The listing builds one solid part. Answer for the finished solid, in the listing's coordinates (mm). A direction names the side the tool comes from. Give positions to 0.01 mm unless a question says otherwise; leave off trailing zeros. Write each loop counter-clockwise with the first axis right and the second up, starting at its lowest first coordinate (ties: lowest second). Pieces come first, ordered by that corner, then holes. Notation, with made-up numbers: (87.25, 71.5) - (114.25, 71.5) arc R19 ccw to (114.25, 87.5) - close; hole circle Ø6 at (67.5, 79.25). An arc over 180 degrees is marked (long way). One line per question, with ' | ' between items. Start each with the question number.
1. Given P1, Ø1, axis at x = -3.5, z = 51.5, coming from the -Y side; P2, Ø6, axis at y = 8.5, z = 20, coming from the +X side; P3, Ø1.5, axis at y = -5, z = 85, coming from the +X side; P4, Ø10, axis at y = -2.5, z = 70.5, coming from the +X side, each flat-ended and moving along its own axis, determine where each tip first touches the part or whether it passes through.
2. Find the intervals of material crossed by L1, parallel to Z at x = -2, y = -2; L2, parallel to Y at x = -3, z = 68; L3, parallel to X at y = 0, z = 31.5, in increasing order. Write a range as from..to.
3. For faces 1 (the face through (-2.4, -1.8, 98)), 2 (the face through (-3, -2, 100)), determine the directions among +Z, -Z, +X, -X, +Y, -Y from which every point of the face is accessible in a straight line to the end or side of a thin tool.
4. The mould has two halves that part along X. Classify faces 3 (the face through (-1.08, 4.88, 46.75)), 4 (the face through (0, 0, 96)), 5 (the face through (0, 0, 0)): +X half, -X half, draft (parallel to the pull), parting line (faces both ways), or undercut.
5. A cutting plane is placed at B-B (x = 0). Determine the outline of the cut face in (y, z), then the cut area to 3 significant figures.
6. A cutting plane is placed at A-A (z = 52). Determine the outline of the cut face in (x, y), then the cut area to 3 significant figures.
Autodesk Inventor part; units mm, degrees
ref_plane "YZ Plane" through (0, 0, 0) normal (1, 0, 0) x (0, 1, 0)
ref_plane "XZ Plane" through (0, 0, 0) normal (0, 1, 0) x (-1, 0, 0)
ref_plane "XY Plane" through (0, 0, 0) normal (0, 0, 1) x (1, 0, 0)
sketch "Sketch1" plane through (0, 0, 0) normal (0, 0, 1) x (1, 0, 0)
  circle A0 centre (0, 0) radius 5
  dimension "Diameter" = 10
extrude "Extrusion1" add sketch "Sketch1" along normal blind 93.8
sketch "Sketch2" plane through (0, 0, 93.8) normal (0, 0, 1) x (1, 0, 0)
  circle A0 centre (0, 0) radius 5
extrude "Extrusion2" add sketch "Sketch2" along normal blind 6.2 draft 45
sketch "Sketch3" plane through (0, 0, 100) normal (0, 0, 1) x (1, 0, 0)
  circle A0 centre (0, 0) radius 11.2
  circle A1 centre (0, 0) radius 3.4641 construction
  line L0 (1.4501, 3.146) -> (3.4495, 0.3172)
  line L1 (3.4495, 0.3172) -> (1.9995, -2.8288)
  line L2 (1.9995, -2.8288) -> (-1.4501, -3.146)
  line L3 (-1.4501, -3.146) -> (-3.4495, -0.3172)
  line L4 (-3.4495, -0.3172) -> (-1.9995, 2.8288)
  line L5 (-1.9995, 2.8288) -> (1.4501, 3.146)
  dimension "Hex_Width" = 6
extrude "Extrusion3" cut sketch "Sketch3" against normal blind 4 contours L0 L1 L2 L3 L4 L5
thread "Thread1"
chamfer "Chamfer2" distance 1 angle 45 1 edges at (-5, 0, 0)
fillet "Fillet1" radius 0.1 1 edges at (-11.2, 0, 100)
equation "\"d10\" = Thread_Length"
equation "\"d13\" = Chamfer"
equation "\"Thread_Length\" = 55"
properties part number "SCREW,FLAT HD,P, 5,M8X1.25X100MM"
Determined:
1) P1: y = -4 | P2: through | P3: x = 2.63 | P4: x = 5
2) L1: 0..96 | L2: -4..4 | L3: -5..5
3) face 1: +Z | face 2: +Z, +X, -X, +Y, -Y
4) face 3: parting line | face 4: undercut | face 5: draft
5) outline: (-11.03, 99.83) - (-5, 93.8) - (-5, 1) - (-4, 0) - (4, 0) - (5, 1) - (5, 93.8) - (11.03, 99.83) arc R0.1 ccw to (10.96, 100) - (3.01, 100) - (3.01, 96) - (-3.01, 96) - (-3.01, 100) - (-10.96, 100) arc R0.1 ccw to start | area: 1,010 mm2
6) outline: circle Ø10 at (0, 0) | area: 78.5 mm2
